Autodesk Inventor part; units mm, degrees
ref_plane "YZ Plane" through (0, 0, 0) normal (1, 0, 0) x (0, 1, 0)
ref_plane "XZ Plane" through (0, 0, 0) normal (0, 1, 0) x (-1, 0, 0)
ref_plane "XY Plane" through (0, 0, 0) normal (0, 0, 1) x (1, 0, 0)
sketch "Sketch1" plane through (0, 0, 0) normal (0, 1, 0) x (-1, 0, 0)
  line L0 (360.8724, 2.8366) -> (-45.5276, 2.8366)
  line L1 (-45.5276, 2.8366) -> (-45.5276, -6.6884)
  line L2 (-45.5276, -6.6884) -> (360.8724, -6.6884)
  line L3 (360.8724, -6.6884) -> (360.8724, 2.8366)
  point P0 (0, 0)
  dimension "d0" = 406.4
  dimension "d1" = 9.525
extrude "Extrusion1" add sketch "Sketch1" along normal blind 3.175
fillet "Fillet1" radius 3.175 2 edges at (-157.6724, 3.175, 2.8366) (-157.6724, 3.175, -6.6884)
properties part number "LED light strip" material "Wood (Oak)"
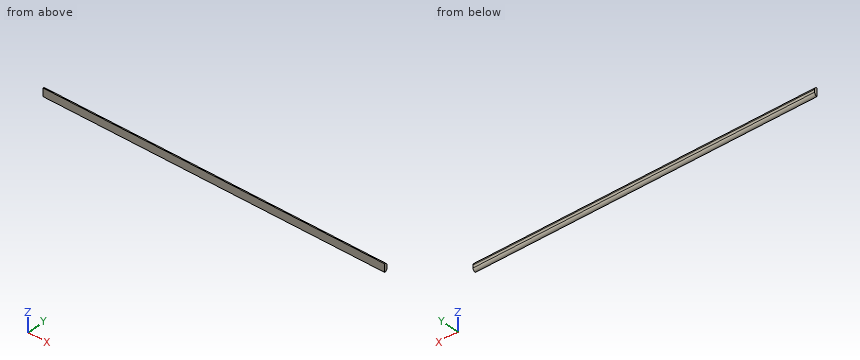
Geometry check sheet. Reference: the model listing, model coordinates, mm. Coordinates: 2 decimals unless noted, no trailing zeros. Order: outer loops, then holes, each group sorted by start corner. A loop starts at its lowest first (then second) coordinate and runs counter-clockwise, first axis right, second up. Notation, with made-up numbers: (87, -27.75) -> (105, -27.75) arc R20 cw to (105, 6.25) -> close; hole circle Ø1 at (2.25, 39). An arc over 180 degrees is marked (long way). Use a Markdown table: item, result. Add a question column.
1. Go/stop test with a flat-tipped pin: pin 1 Ø1.5 at (x, z) = (-36, 1) entering from +Y. Record where the tip stops, or that it passes through.
2. Cross-section at C-C (z = 1.25). Enter the section's corners in (x, y).
3. Material ranges on L1, parallel to Y at x = -13.5, z = 0; L2, parallel to Y at x = -266, z = 0.25; L3, parallel to Z at x = -4.5, y = 0.2, recorded low to high.
4. Cross-section at B-B (y = 1.45). Enter the section's corners in (x, z), and give its area (3 significant figures).
Filled sheet:
| question | item | result |
|---|---|---|
| 1 | pin 1 | y = 3.12 |
| 2 | outline | (-360.87, 0) -> (45.53, 0) -> (45.53, 2.75) -> (-360.87, 2.75) -> close |
| 3 | L1 | 0 to 3.16 |
| 3 | L2 | 0 to 3.12 |
| 3 | L3 | -6.68 to 2.83 |
| 4 | outline | (-360.87, -6.34) -> (45.53, -6.34) -> (45.53, 2.49) -> (-360.87, 2.49) -> close |
| 4 | area | 3,590 mm2 |
